Here's how the part is built. I have some questions about the finished solid (model axes, mm). Face numbers are marked on the shaded views. A direction names the side the tool comes from. Coordinates: 2 decimals unless noted, no trailing zeros. Write each loop counter-clockwise with the first axis right and the second up, starting at its lowest first coordinate (ties: lowest second). Pieces come first, ordered by that corner, then holes.
Autodesk Inventor part; units mm, degrees
ref_plane "Work Plane1" through (-25.7458, -64.4152, -12.319) normal (0, -1, 0) x (0, 0, -1)
ref_plane "Work Plane2" through (0, 0, 0) normal (0, 0, 1) x (1, 0, 0)
ref_plane "YZ Plane" through (0, 0, 0) normal (1, 0, 0) x (0, 1, 0)
ref_plane "Work Plane1" through (-25.7458, -64.4152, -12.319) normal (0, -1, 0) x (0, 0, -1)
ref_plane "Work Plane2" through (0, 0, 0) normal (0, 0, 1) x (1, 0, 0)
sketch "Sketch1" plane through (0, 0, 0) normal (0, 0, 1) x (1, 0, 0)
  line L0 (-0.4093, 18.5158) -> (-5.7433, 18.5158)
  line L1 (-5.7433, -1.2962) -> (-5.7433, 18.5158)
  line L2 (-45.7483, 18.5158) -> (-51.0823, 18.5158)
  line L3 (-45.7483, 18.5158) -> (-45.7483, -1.2962)
  line L4 (-5.7433, 18.5158) -> (4.4167, 18.5158)
  line L5 (4.4167, 18.5158) -> (4.4167, -11.9642)
  line L6 (-45.7483, 18.5158) -> (-55.9083, 18.5158)
  line L7 (-55.9083, 18.5158) -> (-55.9083, -11.9642)
  line L8 (-55.9083, -11.9642) -> (4.4167, -11.9642)
  line L9 (-5.7433, -1.2962) -> (-45.7483, -1.2962)
  point P0 (0, 0)
  dimension "d0" = 10.16
  dimension "d1" = 30.48
  dimension "d2" = 10.16
extrude "Extrusion1" add sketch "Sketch1" along normal blind 1.5875
fillet "Corner Round1" radius 3.175 4 edges at (4.4167, 18.5158, 0.7937) (-5.7433, 18.5158, 0.7937) (-45.7483, 18.5158, 0.7937) (-55.9083, 18.5158, 0.7937)
sketch "Sketch2" plane through (4.4167, -10.3767, 0) normal (0, -1, 0) x (1, 0, 0)
  line L0 (-60.325, 0) -> (0, 0)
  line L1 (0, 0) -> (0, 16.9037)
  line L2 (0, 16.9037) -> (-60.325, 16.9037)
  line L3 (-60.325, 16.9037) -> (-60.325, 0)
edge flange "Flange1" height 16.9037 angle 90 thickness 1.5875 bend radius 1.5875 thickness toward (0, -1, 0) relief straight relief width 1.5875 relief depth 0.7937 edges at (-25.7458, -11.9642, 1.5875) wall of the first edge with corners at (-55.9083, -10.3767, 0) (4.4167, -10.3767, 0) (4.4167, -10.3767, 16.9037) (-55.9083, -10.3767, 16.9037)
bend "Bend1"
corner "Corner1"
sketch "Sketch4" plane through (0, 0, 0) normal (0, 0, -1) x (-1, 0, 0)
  arc A0 (-0.8607, 1.809) -> (-0.8607, 5.4793) centre (1.057, 3.6441) ccw
  arc A1 (-0.8607, 11.7404) -> (-0.8607, 15.4107) centre (1.057, 13.5755) ccw
  arc A2 (52.3523, 15.4107) -> (52.3523, 11.7404) centre (50.4346, 13.5755) ccw
  arc A3 (52.3523, 5.4793) -> (52.3523, 1.809) centre (50.4346, 3.6441) ccw
  arc A4 (52.3523, 1.809) -> (52.3523, 5.4793) centre (50.4346, 3.6441) ccw
  arc A5 (52.3523, 11.7404) -> (52.3523, 15.4107) centre (50.4346, 13.5755) ccw
  arc A6 (-0.8607, 5.4793) -> (-0.8607, 1.809) centre (1.057, 3.6441) ccw
  arc A7 (-0.8607, 15.4107) -> (-0.8607, 11.7404) centre (1.057, 13.5755) ccw
  point P0 (0, 0)
extrude "Extrusion2" cut sketch "Sketch4" against normal up to surface (1.5875 mm away)
ref_plane "Work Plane4" through (4.4167, -10.3767, 3.175) normal (0, 1, 0) x (1, 0, 0)
sketch "Sketch8" plane through (4.4167, -10.3767, 3.175) normal (0, 1, 0) x (1, 0, 0)
  line L0 (12.7, -13.7287) -> (-73.025, -13.7287)
  line L1 (0, 0) -> (-0.1034, -13.7287)
  line L2 (-60.325, 0) -> (0, 0)
  line L3 (-60.325, 0) -> (-60.325, -13.7287)
  line L4 (-3.175, 1.5875) -> (-6.985, 1.5875)
  line L5 (-5.08, 1.5875) -> (-5.08, -6.8643)
  line L6 (-5.08, -6.8643) -> (0, -6.8644)
  line L7 (0, -13.7287) -> (0, 0)
  line L8 (-53.34, 1.5875) -> (-57.15, 1.5875)
  line L9 (-55.245, 1.5875) -> (-55.245, -6.8644)
  point P0 (-4.4167, 3.175)
ref_plane "Work Plane3" through (4.4167, -11.9642, 3.175) normal (0, -1, 0) x (1, 0, 0)
sketch "Sketch9" plane through (4.4167, -11.9642, 3.175) normal (0, -1, 0) x (1, 0, 0)
  line L0 (12.7, 13.7287) -> (-73.025, 13.7287)
  line L1 (0, 13.7287) -> (-60.325, 13.7287)
  line L2 (-60.325, 13.7287) -> (-60.325, 18.8087)
  line L3 (-60.325, 18.8087) -> (0, 18.8087)
  line L4 (0, 18.8087) -> (0, 13.7287)
  line L5 (-60.325, 13.7287) -> (-60.325, 0)
  line L6 (0, 13.7287) -> (0, 0)
  point P0 (-4.4167, -3.175)
  dimension "d57" = 5.08
extrude "Extrusion6" add sketch "Sketch9" against normal blind 1.5875
sketch "Sketch11" plane through (4.4167, -11.9642, 20.3962) normal (0, 0, 1) x (1, 0, 0)
  line L0 (-60.325, 0) -> (0, 0)
  line L1 (0, 0) -> (0, 41.91)
  line L2 (0, 41.91) -> (-60.325, 41.91)
  line L3 (-60.325, 41.91) -> (-60.325, 0)
edge flange "Flange4" height 41.91 angle 90 thickness 1.5875 bend radius 1.5875 thickness toward (0, 0, 1) relief straight relief width 1.5875 relief depth 0.7937 edges at (-25.7458, -10.3767, 21.9837) wall of the first edge with corners at (-55.9083, -11.9642, 20.3962) (4.4167, -11.9642, 20.3962) (4.4167, 29.9458, 20.3962) (-55.9083, 29.9458, 20.3962)
bend "Bend4"
corner "Corner4"
hole "Hole1" at (-0.6633, -10.3767, 10.0393) at (-50.8283, -10.3767, 10.0393) direction (0, -1, 0) diameter 5.1308 end through all
sketch "Sketch12" plane through (4.4167, 29.9458, 20.3962) normal (0, 0, -1) x (-1, 0, 0)
  line L0 (38.354, 0.0162) -> (38.354, -22.9454)
  line L1 (60.325, 0) -> (60.325, -38.735)
  point P0 (4.4167, -29.9458)
  dimension "d65" = 22.9616
  dimension "d66" = 21.971
hole "Hole2" at (-33.9373, 7.0004, 20.3962) direction (0, 0, 1) diameter 28.575 end through all
equation "\"d63\" = Thickness"
equation "\"d72\" = Thickness"
equation "\"d6\" = BendReliefWidth"
equation "\"d7\" = BendReliefDepth"
equation "\"d8\" = MinimumRemnant"
equation "\"d9\" = BendRadius"
equation "\"d12\" = BendRadius"
equation "\"d13\" = CornerReliefSize"
equation "\"d14\" = GapSize"
equation "\"d15\" = JacobiRadiusSize"
equation "\"d47\" = BendReliefWidth"
equation "\"d48\" = BendReliefDepth"
equation "\"d49\" = MinimumRemnant"
equation "\"d50\" = BendRadius"
equation "\"d53\" = BendRadius"
equation "\"d54\" = CornerReliefSize"
equation "\"d55\" = GapSize"
equation "\"d56\" = JacobiRadiusSize"
equation "\"BendRadius\" = Thickness"
equation "\"BendReliefWidth\" = Thickness"
equation "\"BendReliefDepth\" = 0.5 * Thickness"
equation "\"CornerReliefSize\" = 4 * Thickness"
equation "\"MinimumRemnant\" = 2 * Thickness"
equation "\"TransitionRadius\" = BendRadius"
equation "\"JacobiRadiusSize\" = Thickness"
equation "\"GapSize\" = Thickness"
properties part number "HSmountLEFT"
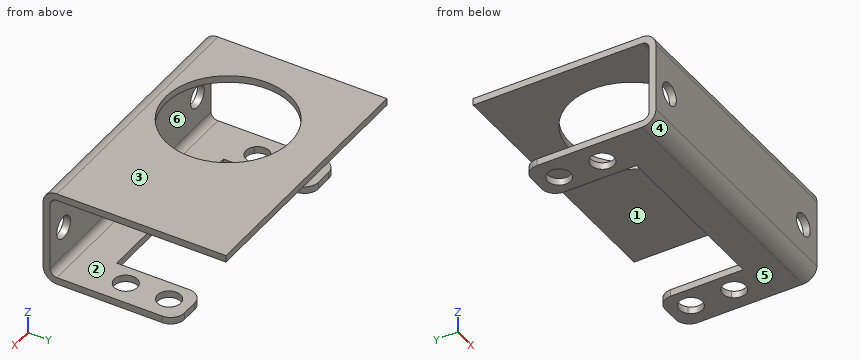
1) Imagine slicing it at D-D on y = -4. Please give me the cut outline in (x, z), then the cut area to 3 significant figures.
Values follow:
outline: (-55.91, 0) - (4.42, 0) - (4.42, 1.59) - (-55.91, 1.59) - close; (-55.91, 20.4) - (-43.05, 20.4) - (-43.05, 21.98) - (-55.91, 21.98) - close; (-24.82, 20.4) - (4.42, 20.4) - (4.42, 21.98) - (-24.82, 21.98) - close
area: 163 mm2
2) I need wall thicknesses on probe 1 along Z at (x, y) = (-13.5, -2); probe 2 along Z at (x, y) = (-11, 4.5); probe 3 along Y at (x, z) = (-7, 18.75). Which ranges of each line are inside material? Lowest first, please.
Values follow:
probe 1: z = 0 to 1.59, 20.4 to 21.98
probe 2: z = 20.4 to 21.98
probe 3: y = -11.96 to -10.38
3) Imagine slicing it at B-B on z = 10.75. Please give me the cut outline in (x, y), then the cut area to 3 significant figures.
Values follow:
outline: (-55.91, -11.96) - (-53.29, -11.96) - (-53.29, -10.38) - (-55.91, -10.38) - close; (-48.36, -11.96) - (-3.13, -11.96) - (-3.13, -10.38) - (-48.36, -10.38) - close; (1.8, -11.96) - (4.42, -11.96) - (4.42, -10.38) - (1.8, -10.38) - close
area: 80.1 mm2
4) Imagine slicing it at A-A on y = 7. Please give me the cut outline in (x, z), then the cut area to 3 significant figures.
Values follow:
outline: (-55.91, 0) - (-45.75, 0) - (-45.75, 1.59) - (-55.91, 1.59) - close; (-55.91, 20.4) - (-48.22, 20.4) - (-48.22, 21.98) - (-55.91, 21.98) - close; (-19.65, 20.4) - (4.42, 20.4) - (4.42, 21.98) - (-19.65, 21.98) - close; (-5.74, 0) - (4.42, 0) - (4.42, 1.59) - (-5.74, 1.59) - close
area: 82.7 mm2
5) On a 3-axis mill with a long thin cutter (end or side, diameter ignored), from which of +Z, -Z, +X, -X, +Y, -Y can I reach the whole of each face in a straight line? I mean the marked faces 5 and 6. Say none if no direction works.
Values follow:
face 5: -Z, +X, -X, +Y, -Y
face 6: +X, -X, +Y
6) Will these pins go through, and if not, where does the flat tip stop? pin 1 (3 mm diameter, centred on x = -1.06, y = 3.64, fed in from -Z); pin 2 (1 mm diameter, centred on x = -46.5, z = 12, fed in from +Y); pin 3 (0.8 mm diameter, centred on x = -1.5, z = 0.5, fed in from +Y).
Values follow:
pin 1: stops at z = 20.4
pin 2: stops at y = -10.38
pin 3: stops at y = 18.52
7) We'd pull the mould along Z, two halves only. Please class the marked faces 1, 2, 3 and 4: pulls with the +Z half, pulls with the -Z half, needs draft (parallel to the pull), parting line crosses it, or undercut.
Values follow:
face 1: undercut
face 2: undercut
face 3: pulls with the +Z half
face 4: pulls with the -Z half
